from build123d import *

# Parameters (mm, degrees)
BOSS_EXTRUDE1_DEPTH = 10
SKETCH3_R           = 5
CUT_EXTRUDE1_DEPTH  = 272.845544381
SKETCH4_R           = 5
CUT_EXTRUDE2_DEPTH  = 272.845544381


with BuildPart() as part:
    # Sketch2 → Boss-Extrude1 (new body)
    with BuildSketch(Plane.XY):
        with BuildLine():
            Line((-260, 0), (260, 0))
            ThreePointArc((260, 0), (267.071067812, 2.928932188), (270, 10))
            Line((270, 10), (270, 20))
            ThreePointArc((270, 20), (267.071067812, 27.071067812), (260, 30))
            Line((260, 30), (-260, 30))
            ThreePointArc((-260, 30), (-267.071067812, 27.071067812), (-270, 20))
            Line((-270, 20), (-270, 10))
            ThreePointArc((-270, 10), (-267.071067812, 2.928932188), (-260, 0))
        make_face()
    extrude(amount=BOSS_EXTRUDE1_DEPTH)

    # Sketch3 → Cut-Extrude1 (cut, through all)
    with BuildSketch(Plane(origin=(0, 0, 0), x_dir=(-1, 0, 0), z_dir=(0, 0, -1))):
        with Locations((254, 15)):
            Circle(SKETCH3_R)
        with Locations((-254, 15)):
            Circle(SKETCH3_R)
    extrude(amount=-CUT_EXTRUDE1_DEPTH, mode=Mode.SUBTRACT)

    # Sketch4 → Cut-Extrude2 (cut, through all)
    with BuildSketch(Plane(origin=(0, 0, 0), x_dir=(-1, 0, 0), z_dir=(0, 0, -1))):
        with Locations((0, 15)):
            Circle(SKETCH4_R)
    extrude(amount=-CUT_EXTRUDE2_DEPTH, mode=Mode.SUBTRACT)


solid = part.part
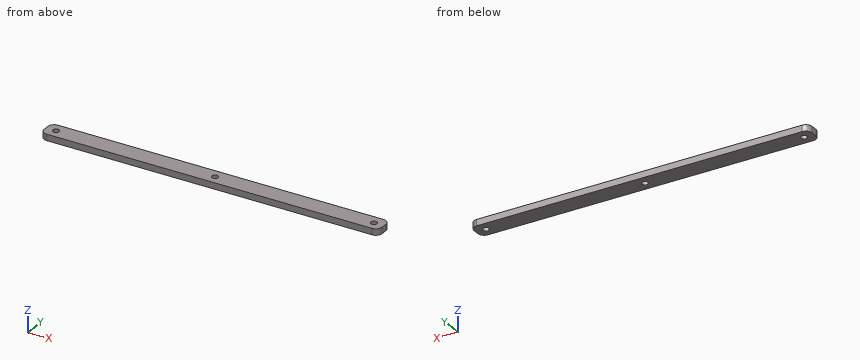
Work out the finished part from the listing and answer in its coordinate system (mm). Give positions to 0.01 mm unless a question says otherwise; leave off trailing zeros. Loops run counter-clockwise (first coordinate to the right, second up) from the corner with the lowest first, then second, coordinate; pieces in that order, holes last. Notation, with made-up numbers: (45.25, 35) -> (101.25, 35) arc R17 cw to (101.25, 68) -> close; hole circle Ø3 at (41.5, -2). An arc over 180 degrees is marked (long way). Use a Markdown table: item, result. Add a question column.
1. Find the intervals of material crossed by probe 1 along X at (y, z) = (13.5, 9); probe 2 along X at (y, z) = (18, 8.75); probe 3 along Y at (x, z) = (254, 6), in increasing order.
2. Section C-C on z = 3.5 is taken. Determine the outline of the cut face in (x, y).
3. Section B-B on x = 254 is taken. Determine the outline of the cut face in (y, z).
4. Section A-A on y = 15 is taken. Determine the outline of the cut face in (x, z), and give its area (3 significant figures).
Results below:
| question | item | result |
|---|---|---|
| 1 | probe 1 | x = -270 to -258.77, -249.23 to -4.77, 4.77 to 249.23, 258.77 to 270 |
| 1 | probe 2 | x = -270 to -258, -250 to -4, 4 to 250, 258 to 270 |
| 1 | probe 3 | y = 0 to 10, 20 to 30 |
| 2 | outline | (-270, 10) arc R10 ccw to (-260, 0) -> (260, 0) arc R10 ccw to (270, 10) -> (270, 20) arc R10 ccw to (260, 30) -> (-260, 30) arc R10 ccw to (-270, 20) -> close; hole circle Ø10 at (-254, 15); hole circle Ø10 at (0, 15); hole circle Ø10 at (254, 15) |
| 3 | outline | (0, 0) -> (10, 0) -> (10, 10) -> (0, 10) -> close; (20, 0) -> (30, 0) -> (30, 10) -> (20, 10) -> close |
| 4 | outline | (-270, 0) -> (-259, 0) -> (-259, 10) -> (-270, 10) -> close; (-249, 0) -> (-5, 0) -> (-5, 10) -> (-249, 10) -> close; (5, 0) -> (249, 0) -> (249, 10) -> (5, 10) -> close; (259, 0) -> (270, 0) -> (270, 10) -> (259, 10) -> close |
| 4 | area | 5,100 mm^2 |
